```python
from build123d import *

# Parameters (mm, degrees)
SKETCH1_W           = 30.48
SKETCH1_H           = 25.4
SKETCH1_R           = 1.651
BOSS_EXTRUDE1_DEPTH = 1.524
SKETCH3_W           = 2.413
SKETCH3_H           = 2.413
BOSS_EXTRUDE2_DEPTH = 2.54
SKETCH4_W           = 0.635
SKETCH4_H           = 0.635
BOSS_EXTRUDE3_DEPTH = 5.715
SKETCH5_W           = 0.635
SKETCH5_H           = 0.635
BOSS_EXTRUDE4_DEPTH = 5.715


with BuildPart() as part:
    # Sketch1 → Boss-Extrude1 (new body)
    with BuildSketch(Plane(origin=(0, 0, 0), x_dir=(1, 0, 0), z_dir=(0, 1, 0))):
        with Locations((15.24, 12.7)):
            Rectangle(SKETCH1_W, SKETCH1_H)
        with Locations((2.54, 22.86)):
            Circle(SKETCH1_R, mode=Mode.SUBTRACT)
        with Locations((27.94, 22.86)):
            Circle(SKETCH1_R, mode=Mode.SUBTRACT)
        with Locations((27.94, 2.54)):
            Circle(SKETCH1_R, mode=Mode.SUBTRACT)
        with Locations((2.54, 2.54)):
            Circle(SKETCH1_R, mode=Mode.SUBTRACT)
    extrude(amount=BOSS_EXTRUDE1_DEPTH)

    # Sketch3 → Boss-Extrude2 (add)
    with BuildSketch(Plane(origin=(0, 0, 0), x_dir=(-1, 0, 0), z_dir=(0, -1, 0))):
        with Locations((-25.3365, 10.16)):
            Rectangle(SKETCH3_W, SKETCH3_H)
        with Locations((-25.3365, 12.7)):
            Rectangle(SKETCH3_W, SKETCH3_H)
        with Locations((-25.3365, 15.24)):
            Rectangle(SKETCH3_W, SKETCH3_H)
        with Locations((-16.51, -0.9525)):
            Rectangle(SKETCH3_W, SKETCH3_H)
        with Locations((-13.97, -0.9525)):
            Rectangle(SKETCH3_W, SKETCH3_H)
        with Locations((-11.43, -0.9525)):
            Rectangle(SKETCH3_W, SKETCH3_H)
        with Locations((-8.89, -0.9525)):
            Rectangle(SKETCH3_W, SKETCH3_H)
    extrude(amount=BOSS_EXTRUDE2_DEPTH)

    # Sketch4 → Boss-Extrude3 (add)
    with BuildSketch(Plane.XY.offset(2.159)):
        with Locations((8.89, -1.27)):
            Rectangle(SKETCH4_W, SKETCH4_H)
        with Locations((11.43, -1.27)):
            Rectangle(SKETCH4_W, SKETCH4_H)
        with Locations((13.97, -1.27)):
            Rectangle(SKETCH4_W, SKETCH4_H)
        with Locations((16.51, -1.27)):
            Rectangle(SKETCH4_W, SKETCH4_H)
    extrude(amount=BOSS_EXTRUDE3_DEPTH)

    # Sketch5 → Boss-Extrude4 (add)
    with BuildSketch(Plane(origin=(26.543, 0, 0), x_dir=(0, 0, -1), z_dir=(1, 0, 0))):
        with Locations((10.16, -1.27)):
            Rectangle(SKETCH5_W, SKETCH5_H)
        with Locations((12.7, -1.27)):
            Rectangle(SKETCH5_W, SKETCH5_H)
        with Locations((15.24, -1.27)):
            Rectangle(SKETCH5_W, SKETCH5_H)
    extrude(amount=BOSS_EXTRUDE4_DEPTH)


solid = part.part
```
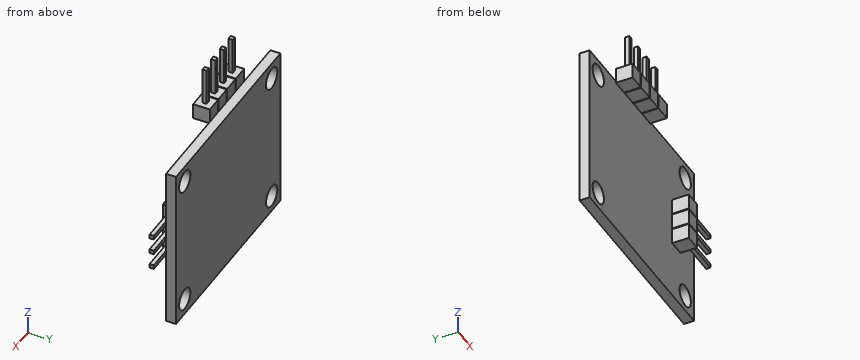
Input: part model. Units: mm. Frame: model coordinates. Give positions to 0.01 mm unless a question says otherwise; leave off trailing zeros. Write each loop counter-clockwise with the first axis right and the second up, starting at its lowest first coordinate (ties: lowest second). Pieces come first, ordered by that corner, then holes. Notation, with made-up numbers: (85.5, -26) - (142.5, -26) arc R12 cw to (142.5, -22) - close; hole circle Ø7 at (11, -30). An arc over 180 degrees is marked (long way). Write item = value, one per line. Start each with the question number.
1) Cut plane A-A (z = 3.5). Return loops of the section in (x, y), and give its area (3 significant figures).
2) Cut plane B-B (x = 2.54). Return loops of the section in (y, z), and give its area (3 significant figures).
3) Pin query (flat end, axial travel): pin 1 (1.2 mm diameter, centred on x = 25.5, y = -0.5, fed in from +Z); pin 2 (3 mm diameter, centred on x = 27.94, z = -2.54, fed in from -Y); pin 3 (1 mm diameter, centred on y = -2, z = -16, fed in from -X); pin 4 (10 mm diameter, centred on x = 7.5, z = -8, fed in from -Y). Return the tip coordinate at first contact, or that it passes through.
4) Cut plane D-D (x = 27.94). Return loops of the section in (y, z).
5) Material intervals for L1, parallel to X at y = 0.7, z = -2.54; L2, parallel to Z at x = 27.94, y = 0.3; L3, parallel to X at y = 0.8, z = -1.5, sorted ascending. Write a range as [from, to].
6) Cut plane C-C (y = 0.75). Return loops of the section in (x, z), and give its area (3 significant figures).
Answers follow:
q1.outline = (8.57, -1.59) - (9.21, -1.59) - (9.21, -0.95) - (8.57, -0.95) - close; (11.11, -1.59) - (11.75, -1.59) - (11.75, -0.95) - (11.11, -0.95) - close; (13.65, -1.59) - (14.29, -1.59) - (14.29, -0.95) - (13.65, -0.95) - close; (16.19, -1.59) - (16.83, -1.59) - (16.83, -0.95) - (16.19, -0.95) - close
q1.area = 1.61 mm^2
q2.outline = (0, -25.4) - (1.52, -25.4) - (1.52, -24.51) - (0, -24.51) - close; (0, -21.21) - (1.52, -21.21) - (1.52, -4.19) - (0, -4.19) - close; (0, -0.89) - (1.52, -0.89) - (1.52, 0) - (0, 0) - close
q2.area = 28.6 mm^2
q3.pin_1 = 0
q3.pin_2 = through
q3.pin_3 = 24.13
q3.pin_4 = 0
q4.outline = (-1.59, -15.56) - (-0.95, -15.56) - (-0.95, -14.92) - (-1.59, -14.92) - close; (-1.59, -13.02) - (-0.95, -13.02) - (-0.95, -12.38) - (-1.59, -12.38) - close; (-1.59, -10.48) - (-0.95, -10.48) - (-0.95, -9.84) - (-1.59, -9.84) - close; (0, -25.4) - (1.52, -25.4) - (1.52, -24.51) - (0, -24.51) - close; (0, -21.21) - (1.52, -21.21) - (1.52, -4.19) - (0, -4.19) - close; (0, -0.89) - (1.52, -0.89) - (1.52, 0) - (0, 0) - close
q5.L1 = [0, 0.89], [4.19, 26.29], [29.59, 30.48]
q5.L2 = [-25.4, -24.51], [-21.21, -4.19], [-0.89, 0]
q5.L3 = [0, 1.26], [3.82, 26.66], [29.22, 30.48]
q6.outline = (0, -25.4) - (30.48, -25.4) - (30.48, 0) - (0, 0) - close; hole circle Ø3.3 at (2.54, -22.86); hole circle Ø3.3 at (2.54, -2.54); hole circle Ø3.3 at (27.94, -22.86); hole circle Ø3.3 at (27.94, -2.54)
q6.area = 740 mm^2
